from build123d import *

# Parameters (mm, degrees)
F0_W     = 184
F0_H     = 82
F0_R     = 26
F1_DEPTH = 5
F0_R_2   = 23
F2_DEPTH = 25
F3_DEPTH = 5
F5_D     = 4.9784


with BuildPart() as f1:
    # F0 (on Front) → F1 (new body)
    with BuildSketch(Plane.XZ):
        Rectangle(F0_W, F0_H)
        with Locations((-51, 0)):
            Circle(F0_R, mode=Mode.SUBTRACT)
        with Locations((51, 0)):
            Circle(F0_R, mode=Mode.SUBTRACT)
    extrude(amount=F1_DEPTH)

    # F0 (on Front) → F2 (join)
    with BuildSketch(Plane.XZ):
        with Locations((-51, 0)):
            Circle(F0_R)
        with Locations((-51, 0)):
            Circle(F0_R_2, mode=Mode.SUBTRACT)
        with Locations((51, 0)):
            Circle(F0_R)
        with Locations((51, 0)):
            Circle(F0_R_2, mode=Mode.SUBTRACT)
    extrude(amount=-F2_DEPTH)

    # F0 (on Front) → F3 (join)
    with BuildSketch(Plane.XZ):
        with Locations((-51, 0)):
            Circle(F0_R)
        with Locations((-51, 0)):
            Circle(F0_R_2, mode=Mode.SUBTRACT)
        with Locations((51, 0)):
            Circle(F0_R)
        with Locations((51, 0)):
            Circle(F0_R_2, mode=Mode.SUBTRACT)
    extrude(amount=F3_DEPTH)

    # F5 (through all)
    with Locations(Plane(origin=(0, 0, 0), x_dir=(1, 0, 0), z_dir=(0, 1, 0))):
        with Locations((-83, -32), (0, -32), (83, -32), (83, 32), (0, 32), (-83, 32)):
            Hole(F5_D / 2)


solid = f1.part
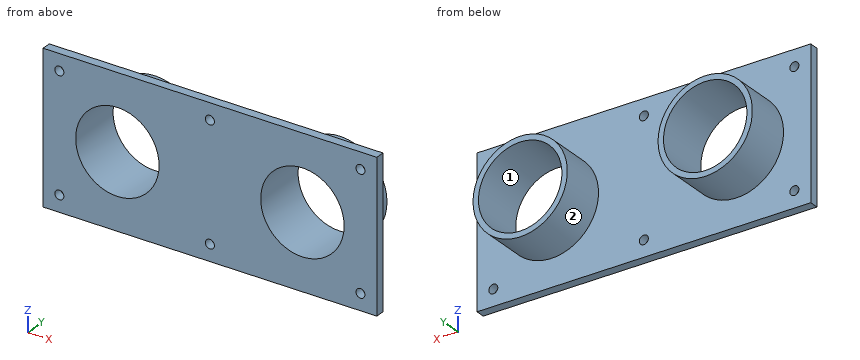
Here's how the part is built. I have some questions about the finished solid (model axes, mm). Face numbers are marked on the shaded views. A direction names the side the tool comes from. Give positions to 0.01 mm unless a question says otherwise; leave off trailing zeros. Order: outer loops, then holes, each group sorted by start corner. A loop starts at its lowest first (then second) coordinate and runs counter-clockwise, first axis right, second up. Notation, with made-up numbers: (13, -19) -> (50, -19) arc R34 cw to (50, 11) -> close; hole circle Ø11 at (21, 41.5). An arc over 180 degrees is marked (long way). Use a Markdown table: item, result. Add a question column.
Item 1: Imagine slicing it at B-B on x = 0. Please give me the cut outline in (y, z), plus the area to 3 significant figures.
Item 2: Imagine slicing it at A-A on z = 32. Please give me the cut outline in (x, y).
Item 3: Imagine slicing it at D-D on y = 22. Please give me the cut outline in (x, z).
Item 4: Imagine slicing it at C-C on y = -2. Give the number of separate pieces and of enclosed holes in the cut face, plus the area to 3 significant figures.
Item 5: Will these pins go through, and if not, where does the flat tip stop? pin 1 (4 mm diameter, centred on x = 62, y = 6.5, fed in from -Z); pin 2 (1.5 mm diameter, centred on x = 73, y = 16, fed in from +Z); pin 3 (1 mm diameter, centred on y = 21, z = 18.5, fed in from +X).
Item 6: I need wall thicknesses on line 1 (Z direction, x = 83, y = -3.45); line 2 (X direction, y = -2.8, z = -32); line 3 (X direction, y = 17, z = 1). Which ranges of each line are inside material? Lowest first, please.
Item 7: For the marked faces 1 and 2, which set-ups out of +Z, -Z, +X, -X, +Y, -Y let a thin tool reach every point of the face, with its end or its side?
Data:
| question | item | result |
|---|---|---|
| 1 | outline | (-5, -41) -> (0, -41) -> (0, -34.49) -> (-5, -34.49) -> close; (-5, -29.51) -> (0, -29.51) -> (0, 29.51) -> (-5, 29.51) -> close; (-5, 34.49) -> (0, 34.49) -> (0, 41) -> (-5, 41) -> close |
| 1 | area | 360 mm² |
| 2 | outline | (-92, -5) -> (-85.49, -5) -> (-85.49, 0) -> (-92, 0) -> close; (-80.51, -5) -> (-2.49, -5) -> (-2.49, 0) -> (-80.51, 0) -> close; (2.49, -5) -> (80.51, -5) -> (80.51, 0) -> (2.49, 0) -> close; (85.49, -5) -> (92, -5) -> (92, 0) -> (85.49, 0) -> close |
| 3 | outline | circle Ø52 at (-51, 0); circle Ø52 at (51, 0); hole circle Ø46 at (-51, 0); hole circle Ø46 at (51, 0) |
| 4 | separate pieces | 1 |
| 4 | enclosed holes | 8 |
| 4 | area | 11,600 mm² |
| 5 | pin 1 | stops at z = -24.39 |
| 5 | pin 2 | stops at z = 14.98 |
| 5 | pin 3 | stops at x = 69.76 |
| 6 | line 1 | z = -41 to -34.49, -29.51 to 29.51, 34.49 to 41 |
| 6 | line 2 | x = -92 to -85.49, -80.51 to -2.49, 2.49 to 80.51, 85.49 to 92 |
| 6 | line 3 | x = -76.98 to -73.98, -28.02 to -25.02, 25.02 to 28.02, 73.98 to 76.98 |
| 7 | face 1 | +Y, -Y |
| 7 | face 2 | +Y |
